from build123d import *

# Parameters (mm, degrees)
SKETCH1_R           = 1.6383
BOSS_EXTRUDE1_DEPTH = 1.575
CUT_EXTRUDE1_DEPTH  = 2.54
SKETCH15_R          = 1.524
CUT_EXTRUDE5_DEPTH  = 1.575


with BuildPart() as part:
    # Sketch1 → Boss-Extrude1 (new body)
    with BuildSketch(Plane(origin=(0, 0, 0), x_dir=(1, 0, 0), z_dir=(0, 1, 0))):
        with BuildLine():
            Line((-38.395, 30), (-42.73, 30))
            ThreePointArc((-42.73, 30), (-43.628025612, 30.371974388), (-44, 31.27))
            Line((-44, 31.27), (-44, 45))
            ThreePointArc((-44, 45), (-43.414213562, 46.414213562), (-42, 47))
            Line((-42, 47), (42, 47))
            ThreePointArc((42, 47), (43.414213562, 46.414213562), (44, 45))
            Line((44, 45), (44, 32))
            ThreePointArc((44, 32), (43.414213562, 30.585786438), (42, 30))
            Line((42, 30), (38.395, 30))
            ThreePointArc((38.395, 30), (37.496974388, 29.628025612), (37.125, 28.73))
            Line((37.125, 28.73), (37.125, -35.73))
            ThreePointArc((37.125, -35.73), (37.496974388, -36.628025612), (38.395, -37))
            Line((38.395, -37), (42, -37))
            ThreePointArc((42, -37), (43.414213562, -37.585786438), (44, -39))
            Line((44, -39), (44, -47))
            Line((44, -47), (-42, -47))
            ThreePointArc((-42, -47), (-43.414213562, -46.414213562), (-44, -45))
            Line((-44, -45), (-44, -38.977))
            ThreePointArc((-44, -38.977), (-43.40945979, -37.574276641), (-42, -37))
            Line((-42, -37), (-38.395, -37))
            ThreePointArc((-38.395, -37), (-37.496974388, -36.628025612), (-37.125, -35.73))
            Line((-37.125, -35.73), (-37.125, 28.73))
            ThreePointArc((-37.125, 28.73), (-37.496974388, 29.628025612), (-38.395, 30))
        make_face()
        with Locations(Location((40, 43.5, 0), (0, 0, 270))):
            Circle(SKETCH1_R, mode=Mode.SUBTRACT)
        with Locations(Location((-40, 43.5, 0), (0, 0, 270))):
            Circle(SKETCH1_R, mode=Mode.SUBTRACT)
        with Locations(Location((-37.6, -42.1, 0), (0, 0, 270))):
            Circle(SKETCH1_R, mode=Mode.SUBTRACT)
        with Locations(Location((36.1, -42.1, 0), (0, 0, 270))):
            Circle(SKETCH1_R, mode=Mode.SUBTRACT)
        Polygon((23, -31.5), (-23, -31.5), (-23, -8.5), (-12.5, -8.5), (-12.5, 35), (12.5, 35), (12.5, -8.5), (23, -8.5), align=None, mode=Mode.SUBTRACT)
    extrude(amount=BOSS_EXTRUDE1_DEPTH)

    # Sketch2 → Cut-Extrude1 (cut)
    with BuildSketch(Plane(origin=(0, 1.575, 0), x_dir=(1, 0, 0), z_dir=(0, 1, 0))):
        Polygon((-12.5, 18.255354416), (-30.026, 18.255354416), (-30.026, 47), (30.026, 47), (30.026, 18.255354416), (12.5, 18.255354416), (12.5, 35), (-12.5, 35), align=None)
    extrude(amount=-CUT_EXTRUDE1_DEPTH, mode=Mode.SUBTRACT)

    # Sketch15 → Cut-Extrude5 (cut)
    with BuildSketch(Plane(origin=(0, 1.575, 0), x_dir=(1, 0, 0), z_dir=(0, 1, 0))):
        with Locations(Location((-36.376, 36.35, 0), (0, 0, 270))):
            Circle(SKETCH15_R)
        with Locations(Location((36.376, 36.332, 0), (0, 0, 270))):
            Circle(SKETCH15_R)
    extrude(amount=-CUT_EXTRUDE5_DEPTH, mode=Mode.SUBTRACT)


solid = part.part
Part model, mm, in its own coordinate system. A direction names the side the tool comes from. Coordinates: 2 decimals unless noted, no trailing zeros. Loops run counter-clockwise (first coordinate to the right, second up) from the corner with the lowest first, then second, coordinate; pieces in that order, holes last. Notation, with made-up numbers: (-28.75, 6.5) - (23.25, 6.5) arc R34 ccw to (23.25, 40.5) - close; hole circle Ø1 at (57, 51). An arc over 180 degrees is marked (long way). Write each question's results on one line, items separated by ' | '. Start each with the question number.
Q1. Slice it at A-A on z = -43.5. Give the cut face in (x, y) (3 decimals), and give its area (3 significant figures).
Q2. Which spindle directions (+Z, -Z, +X, -X, +Y, -Y) get a long thin tool onto all of the face, cutting with end or side? Do faces 1 (the cylindrical face through (43.43, 0.78, -30.6)), 2 (the cylindrical face through (34.888, 0.799, -36.662)). Say none if no direction does.
Q3. Slice it at C-C on z = -13. Give the cut face in (x, y) (3 decimals), and give its area (3 significant figures).
Q4. Slice it at B-B on x = -21. Give the cut face in (y, z) (3 decimals).
Q5. Probe line 1 along X through (y, z) = (1.15, 42.1); line 2 along X through (y, z) = (0.45, -36.35); line 3 along X through (y, z) = (0.7, 23) (3 decimals). List the from-to ranges inside material, lowest first.
Q6. Slice it at D-D on z = 42.1. Give the cut face in (x, y) (3 decimals).
Q7. Drop flat-ended pins along their axis: pin 1 Ø0.8 at (x, y) = (21, 0.5) entering from -Z; pin 2 Ø5 at (x, z) = (-29.5, 11.5) entering from -Y; pin 3 Ø0.8 at (y, z) = (1, 22.5) entering from -X (3 decimals). Give the stop position or say it passes through.
Q8. Two-plate mould, pull along X, no slides. Class faces 3 (the cylindrical face through (43.4, 0.78, 37.57)), 4 (the cylindrical face through (-43.43, 0.78, -46.4)), 5 (the cylindrical face through (36.172, 0.776, 40.463)), 6 (the flat face through (13, 1.575, 7)): +X half, -X half, draft (parallel to the pull), parting line (faces both ways), or undercut.
Answer:
1) outline: (-44, 0) - (-41.638, 0) - (-41.638, 1.575) - (-44, 1.575) - close; (-38.362, 0) - (-30.026, 0) - (-30.026, 1.575) - (-38.362, 1.575) - close; (30.026, 0) - (38.362, 0) - (38.362, 1.575) - (30.026, 1.575) - close; (41.638, 0) - (44, 0) - (44, 1.575) - (41.638, 1.575) - close | area: 33.7 mm2
2) face 1: +X, +Y, -Y | face 2: +Y, -Y
3) outline: (-37.125, 0) - (-12.5, 0) - (-12.5, 1.575) - (-37.125, 1.575) - close; (12.5, 0) - (37.125, 0) - (37.125, 1.575) - (12.5, 1.575) - close | area: 77.6 mm2
4) outline: (0, -18.255) - (1.575, -18.255) - (1.575, 8.5) - (0, 8.5) - close; (0, 31.5) - (1.575, 31.5) - (1.575, 47) - (0, 47) - close
5) line 1: x = -44 to -39.24, -35.96 to 34.46, 37.74 to 44 | line 2: x = -44 to -37.9, -34.85 to -30.03, 30.03 to 34.85, 37.9 to 44 | line 3: x = -37.125 to -23, 23 to 37.125
6) outline: (-44, 0) - (-39.238, 0) - (-39.238, 1.575) - (-44, 1.575) - close; (-35.962, 0) - (34.462, 0) - (34.462, 1.575) - (-35.962, 1.575) - close; (37.738, 0) - (44, 0) - (44, 1.575) - (37.738, 1.575) - close
7) pin 1: stops at z = -18.26 | pin 2: stops at y = 0 | pin 3: stops at x = -37.125
8) face 3: +X half | face 4: -X half | face 5: undercut | face 6: draft
